Source: CAD feature listing. Evaluate the final solid. Frame: model axes, mm. Give positions to 0.01 mm unless a question says otherwise; leave off trailing zeros. Write each loop counter-clockwise with the first axis right and the second up, starting at its lowest first coordinate (ties: lowest second). Pieces come first, ordered by that corner, then holes. Notation, with made-up numbers: (66, 27) -> (114, 27) arc R19 ccw to (114, 34) -> close; hole circle Ø3 at (28.25, -9). An arc over 180 degrees is marked (long way). Answer as a JSON object with one key per item and string values. Group by question number.
Item 1: Ray query, probe 1 along Y at (x, z) = (0, 1.95); probe 2 along Z at (x, y) = (-6.25, -8); probe 3 along Y at (x, z) = (0, 3.05). Return the intervals inside material, ascending. Write a range as from..to.
Item 2: Section query C-C on x = -9.25. Return the cut outline in (y, z), plus the area to 3 significant figures.
Item 3: Pull-direction query (X, two-part tool) for faces 1 (the face through (0, -2, 0)), 2 (the face through (0.108, -0.488, 1.972)), 3 (the face through (-1.5, 11.4, 1)); classes: pulls with the +X half, pulls with the -X half, needs draft (parallel to the pull), parting line crosses it, or undercut.
Item 4: Section query A-A on z = 1.6. Return the cut outline in (x, y).
Item 5: First-contact query: pin 1 Ø2 at (y, z) = (-8.5, 2.5) entering from +X; pin 2 Ø2 at (x, z) = (-1.5, 1.5) entering from +Y. Flat tips, straight axial feed; report the tip coordinate or a pass-through.
Item 6: Section query B-B on y = 9.5. Return the cut outline in (x, z), plus the area to 3 significant figures.
from build123d import *

# Parameters (mm, degrees)
ESQUISSE1_R             = 11.5
BOSS_EXTRU_1_DEPTH      = 2
ESQUISSE6_RX            = 6
ESQUISSE6_RY            = 2.5
BOSS_EXTRU_5_DEPTH      = 2
ESQUISSE7_R             = 0.5
ENL_V_MAT_EXTRU_1_DEPTH = 17.748134224


with BuildPart() as part:
    # Esquisse1 → Boss.-Extru.1 (new body)
    with BuildSketch(Plane.XY):
        Circle(ESQUISSE1_R)
    extrude(amount=BOSS_EXTRU_1_DEPTH)

    # Esquisse6 → Boss.-Extru.5 (add)
    with BuildSketch(Plane.XY.offset(2)):
        with Locations((0, 0)):
            Ellipse(ESQUISSE6_RX, ESQUISSE6_RY)
    extrude(amount=BOSS_EXTRU_5_DEPTH)

    # Esquisse7 → Enlèv. mat.-Extru.1 (cut, through all)
    with BuildSketch(Plane(origin=(0, 0, 0), x_dir=(-1, 0, 0), z_dir=(0, 0, -1))):
        Circle(ESQUISSE7_R)
    extrude(amount=-ENL_V_MAT_EXTRU_1_DEPTH, mode=Mode.SUBTRACT)


solid = part.part
Worked answers:
{
 "1": {"probe 1": "-11.5..-0.5, 0.5..11.5", "probe 2": "0..2", "probe 3": "-2.5..-0.5, 0.5..2.5"},
 "2": {"outline": "(-6.83, 0) -> (6.83, 0) -> (6.83, 2) -> (-6.83, 2) -> close", "area": "27.3 mm^2"},
 "3": {"face 1": "needs draft", "face 2": "undercut", "face 3": "parting line crosses it"},
 "4": {"outline": "circle Ø23 at (0, 0); hole circle Ø1 at (0, 0)"},
 "5": {"pin 1": "x = 8.6", "pin 2": "y = 11.49"},
 "6": {"outline": "(-6.48, 0) -> (6.48, 0) -> (6.48, 2) -> (-6.48, 2) -> close", "area": "25.9 mm^2"}
}
